from build123d import *

# Parameters (mm, degrees)
F0_R      = 25
F1_DEPTH  = 10
F2_W      = 60
F2_H      = 56.883122
F1_FACE_R = 25
F3_DEPTH  = 29.8
F4_R      = 15
F5_DEPTH  = 47.7


with BuildPart() as f1:
    # F0 (on Top) → F1 (new body)
    with BuildSketch(Plane.XY):
        Circle(F0_R)
    extrude(amount=F1_DEPTH)

    # F2 (on Top) + F1_face (on face) → F3 (join)
    with BuildSketch(Plane.XY):
        Rectangle(F2_W, F2_H)
    with BuildSketch(Plane.XY.offset(10)):
        Circle(F1_FACE_R)
    extrude(amount=-F3_DEPTH)

    # F4 (on face) → F5 (cut)
    with BuildSketch(Plane.XY.offset(10)):
        Circle(F4_R)
    extrude(amount=-F5_DEPTH, mode=Mode.SUBTRACT)


solid = f1.part
Could you check a few things on this model? Use its own coordinates, in mm. A direction names the side the tool comes from. Give positions to 0.01 mm unless a question says otherwise; leave off trailing zeros. Order: outer loops, then holes, each group sorted by start corner. A loop starts at its lowest first (then second) coordinate and runs counter-clockwise, first axis right, second up. Notation, with made-up numbers: (43.25, 20.25) - (79.25, 20.25) arc R26 cw to (79.25, 43.25) - close; hole circle Ø7 at (-13, 67). An arc over 180 degrees is marked (long way). One line per item, written item: value. Start each with the question number.
1. If I drill on probe 1 along Y at (x, z) = (0, -12.5); probe 2 along Z at (x, y) = (-21.5, -18); probe 3 along X at (y, z) = (-8, -18.5), over which ranges is the centre line in solid material (lowest first)?
2. Imagine slicing it at D-D on y = 20. List the corners of the cut face in (x, z) for me.
3. Imagine slicing it at C-C on z = -13.5. List the corners of the cut face in (x, y) for me.
4. Thinking about a two-plate mould opening in Y: for faces 1 (the face through (0, -28.442, -15)), 2 (the face through (30, 0, -15)), 3 (the face through (0, 28.442, -15)), 4 (the face through (-14.985, 0.66, -9.621)), which applies, +Y half, -Y half, draft (parallel to the pull), parting line (faces both ways), or undercut?
5. Imagine slicing it at A-A on y = 0. List the corners of the cut face in (x, z) for me.
6. For P1, Ø1.5, axis at y = 8, z = 5, coming from the +X side, with a flat end and sliding along its axis, tell me the tip position at first contact or that it passes through.
7. Imagine slicing it at B-B on x = 0. List the corners of the cut face in (y, z) for me.
8. For faces 5 (the face through (-14, 7, -29.8)), 6 (the face through (0, 26, 0)), which set-ups out of +Z, -Z, +X, -X, +Y, -Y let a thin tool reach every point of the face, with its end or its side?
Values:
1. probe 1: -28.44 to -15, 15 to 28.44
1. probe 2: -29.8 to 0
1. probe 3: -30 to -12.69, 12.69 to 30
2. outline: (-30, -29.8) - (30, -29.8) - (30, 0) - (15, 0) - (15, 10) - (-15, 10) - (-15, 0) - (-30, 0) - close
3. outline: (-30, -28.44) - (30, -28.44) - (30, 28.44) - (-30, 28.44) - close; hole circle Ø30 at (0, 0)
4. face 1: -Y half
4. face 2: draft
4. face 3: +Y half
4. face 4: undercut
5. outline: (-30, -29.8) - (-15, -29.8) - (-15, 10) - (-25, 10) - (-25, 0) - (-30, 0) - close; (15, -29.8) - (30, -29.8) - (30, 0) - (25, 0) - (25, 10) - (15, 10) - close
6. P1: x = 23.93
7. outline: (-28.44, -29.8) - (-15, -29.8) - (-15, 10) - (-25, 10) - (-25, 0) - (-28.44, 0) - close; (15, -29.8) - (28.44, -29.8) - (28.44, 0) - (25, 0) - (25, 10) - (15, 10) - close
8. face 5: -Z, +X, -X, +Y, -Y
8. face 6: +Z
